from build123d import *

# Parameters (mm, degrees)
FILLET_R        = 6
FILLET001_R     = 3.5
POCKET_DEPTH    = 1
POCKET001_DEPTH = 8
SKETCH004_R     = 1.5
POCKET002_DEPTH = 5
POCKET003_DEPTH = 5
SKETCH006_R     = 2
POCKET004_DEPTH = 5


with BuildPart() as part:
    # Sketch → AdditiveLoft section 0
    with BuildSketch(Plane.XY):
        with BuildLine():
            Line((-114.5, 111), (114.5, 111))
            ThreePointArc((109.5, -20), (112.998546, 45.461888), (114.5, 111))
            Line((109.5, -20), (-109.5, -20))
            ThreePointArc((-114.5, 111), (-112.998546, 45.461888), (-109.5, -20))
        make_face()
    # Sketch001 → AdditiveLoft section 1
    with BuildSketch(Plane.XY.offset(-12.5)):
        with BuildLine():
            Line((-113.5, 110), (113.5, 110))
            ThreePointArc((108.5, -19), (111.9985, 45.461298), (113.5, 110))
            Line((108.5, -19), (-108.5, -19))
            ThreePointArc((-113.5, 110), (-111.9985, 45.461298), (-108.5, -19))
        make_face()
    loft()

    # Fillet
    fillet_edges = [part.edges().sort_by_distance(p)[0] for p in [
        (-114, 110.5, -6.25),
        (114, 110.5, -6.25),
    ]]
    fillet(fillet_edges, radius=FILLET_R)

    # Fillet001
    fillet001_edges = [part.edges().sort_by_distance(p)[0] for p in [
        (-109, -19.5, -6.25),
        (109, -19.5, -6.25),
    ]]
    fillet(fillet001_edges, radius=FILLET001_R)

    # Sketch002 (on Face1 of Fillet001) → Pocket (cut)
    with BuildSketch(Plane.XY):
        with BuildLine():
            Line((-88.75, 106), (88.75, 106))
            ThreePointArc((96.75, 98), (94.406854, 103.656854), (88.75, 106))
            Line((96.75, 98), (96.75, 3))
            ThreePointArc((88.75, -5), (94.406854, -2.656854), (96.75, 3))
            Line((88.75, -5), (-88.75, -5))
            ThreePointArc((-96.75, 3), (-94.406854, -2.656854), (-88.75, -5))
            Line((-96.75, 3), (-96.75, 98))
            ThreePointArc((-88.75, 106), (-94.406854, 103.656854), (-96.75, 98))
        make_face()
    extrude(amount=-POCKET_DEPTH, mode=Mode.SUBTRACT)

    # Sketch003 (on Face19 of Pocket) → Pocket001 (cut)
    with BuildSketch(Plane.XY.offset(-1)):
        with BuildLine():
            Line((-87.75, 104), (87.75, 104))
            ThreePointArc((94.75, 97), (92.699747, 101.949747), (87.75, 104))
            Line((94.75, 97), (94.75, 4))
            ThreePointArc((87.75, -3), (92.699747, -0.949747), (94.75, 4))
            Line((87.75, -3), (-87.75, -3))
            ThreePointArc((-94.75, 4), (-92.699747, -0.949747), (-87.75, -3))
            Line((-94.75, 4), (-94.75, 97))
            ThreePointArc((-87.75, 104), (-92.699747, 101.949747), (-94.75, 97))
        make_face()
    extrude(amount=-POCKET001_DEPTH, mode=Mode.SUBTRACT)

    # Sketch004 (on Face28 of Pocket001) → Pocket002 (cut)
    with BuildSketch(Plane.XY.offset(-9)):
        with Locations((-61.34, 84.42)):
            Circle(SKETCH004_R)
        with Locations((64.86, 84.42)):
            Circle(SKETCH004_R)
        with Locations((64.86, 18.77)):
            Circle(SKETCH004_R)
        with Locations((-61.34, 18.77)):
            Circle(SKETCH004_R)
    extrude(amount=-POCKET002_DEPTH, mode=Mode.SUBTRACT)

    # Sketch005 (on Face32 of Pocket002) → Pocket003 (cut)
    with BuildSketch(Plane.XY.offset(-9)):
        with BuildLine():
            Line((-51.75, 99), (51.75, 99))
            ThreePointArc((54.75, 96), (53.87132, 98.12132), (51.75, 99))
            Line((54.75, 96), (54.75, 5))
            ThreePointArc((51.75, 2), (53.87132, 2.87868), (54.75, 5))
            Line((51.75, 2), (-51.75, 2))
            ThreePointArc((-54.75, 5), (-53.87132, 2.87868), (-51.75, 2))
            Line((-54.75, 5), (-54.75, 96))
            ThreePointArc((-51.75, 99), (-53.87132, 98.12132), (-54.75, 96))
        make_face()
    extrude(amount=-POCKET003_DEPTH, mode=Mode.SUBTRACT)

    # Sketch006 (on Face18 of Pocket003) → Pocket004 (cut)
    with BuildSketch(Plane(origin=(0, 0, -12.5), x_dir=(1, 0, 0), z_dir=(0, 0, -1))):
        with Locations((97.5, -86)):
            Circle(SKETCH006_R)
        with Locations((97.5, -2)):
            Circle(SKETCH006_R)
        with Locations((-97.5, -2)):
            Circle(SKETCH006_R)
        with Locations((-97.5, -86)):
            Circle(SKETCH006_R)
    extrude(amount=-POCKET004_DEPTH, mode=Mode.SUBTRACT)


solid = part.part
Model file for the job. Use its own axes, mm. A direction names the side the tool comes from. Round coordinates to 2 decimals unless told otherwise and drop trailing zeros.
(1) 3-axis set-ups, long thin cutter, end or side, ignore diameter. For faces 3 (the face through (97, 86, -7.5)), 4 (the face through (94.75, 51, -5)), 5 (the face through (-7, -1, -12.5)): which of +Z, -Z, +X, -X, +Y, -Y reach the whole face in a straight line?
(2) Pin check, flat tips, straight feed: pin 1 (12 mm diameter, centred on x = -59.5, y = 96, fed in from +Z); pin 2 (2 mm diameter, centred on y = 83.5, z = -2.5, fed in from -X); pin 3 (3 mm diameter, centred on y = 69.5, z = -10.5, fed in from -X). Stop position of each tip, or through.
(3) Pull direction X, two halves, no side cores. Call faces 1 (the face through (64, 51, -9)), 2 (the face through (-6, -8, 0)): released by +X, released by -X, zero draft, split by the parting line, or undercut.
(4) Drill centre lines: line 1 (Y direction, x = -97.5, z = -8.95); line 2 (X direction, y = 84.42, z = -11.25); line 3 (Z direction, x = -61, y = 92). Where is each one in solid material? Low to high.
Verdict:
1. face 3: -Z
1. face 4: +Z
1. face 5: -Z, +X, -X, +Y, -Y
2. pin 1: stops at z = -9
2. pin 2: stops at x = -114
2. pin 3: stops at x = -113.08
3. face 1: undercut
3. face 2: zero draft
4. line 1: y = -19.28 to 0, 4 to 84, 88 to 110.28
4. line 2: x = -113.24 to -98.73, -96.27 to -62.84, -59.84 to -54.75, 54.75 to 63.36, 66.36 to 96.27, 98.73 to 113.24
4. line 3: z = -12.5 to -9
